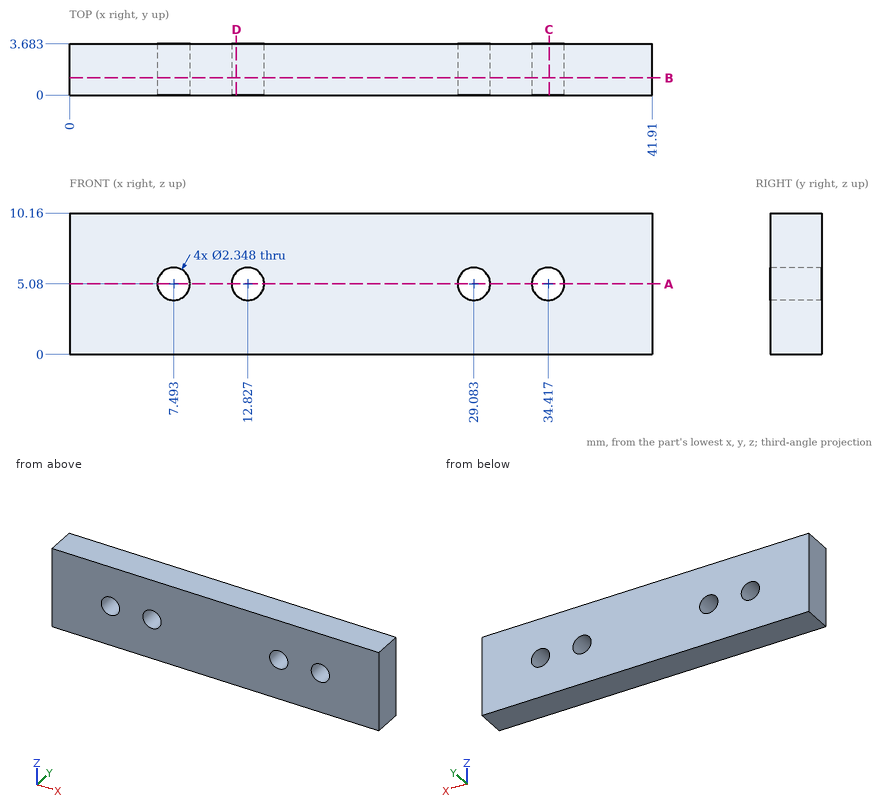
Answer from the drawing. Dimensions are ordinates in mm from the lowest x, y and z of the part. Coordinates: 2 decimals unless noted, no trailing zeros. Loops run counter-clockwise (first coordinate to the right, second up) from the corner with the lowest first, then second, coordinate; pieces in that order, holes last.
1) A flat-ended cylindrical pin translates along its axis: pin 1 (1.9 mm diameter, centred on x = 34.417, z = 5.08, fed in from +Y). Find the tip coordinate at first contact, or state that the pin passes through.
Results:
pin 1: passes through
2) Section A-A (z = 5.08) is taken. Give the vertices of the cut face in (x, y).
Results:
outline: (0, 0) - (6.32, 0) - (6.32, 3.68) - (0, 3.68) - close; (8.67, 0) - (11.65, 0) - (11.65, 3.68) - (8.67, 3.68) - close; (14, 0) - (27.91, 0) - (27.91, 3.68) - (14, 3.68) - close; (30.26, 0) - (33.24, 0) - (33.24, 3.68) - (30.26, 3.68) - close; (35.59, 0) - (41.91, 0) - (41.91, 3.68) - (35.59, 3.68) - close
3) Section D-D (x = 12) is taken. Give the vertices of the cut face in (y, z), plus the area to 3 significant figures.
Results:
outline: (0, 0) - (3.68, 0) - (3.68, 4.25) - (0, 4.25) - close; (0, 5.91) - (3.68, 5.91) - (3.68, 10.16) - (0, 10.16) - close
area: 31.3 mm2
4) Consider probe 1 along X at (y, z) = (1, 5); probe 2 along Z at (x, y) = (7.5, 3.3); probe 3 along X at (y, z) = (1.85, 5.5). Determine where each line is inside the solid, lowest interval first.
Results:
probe 1: x = 0 to 6.32, 8.66 to 11.66, 14 to 27.91, 30.25 to 33.25, 35.59 to 41.91
probe 2: z = 0 to 3.91, 6.25 to 10.16
probe 3: x = 0 to 6.4, 8.59 to 11.73, 13.92 to 27.99, 30.18 to 33.32, 35.51 to 41.91
5) Section C-C (x = 34.5) is taken. Give the vertices of the cut face in (y, z).
Results:
outline: (0, 0) - (3.68, 0) - (3.68, 3.91) - (0, 3.91) - close; (0, 6.25) - (3.68, 6.25) - (3.68, 10.16) - (0, 10.16) - close
6) Section B-B (y = 1.25) is taken. Give the vertices of the cut face in (x, z), plus the area to 4 significant figures.
Results:
outline: (0, 0) - (41.91, 0) - (41.91, 10.16) - (0, 10.16) - close; hole circle Ø2.35 at (7.49, 5.08); hole circle Ø2.35 at (12.83, 5.08); hole circle Ø2.35 at (29.08, 5.08); hole circle Ø2.35 at (34.42, 5.08)
area: 408.5 mm2
